```python
from build123d import *

# Parameters (mm, degrees)
F1_DEPTH = 50.8
F2_R     = 50.8
F3_R     = 5.08


with BuildPart() as f1:
    # F0 (on Top) → F1 (new body)
    with BuildSketch(Plane.XY):
        Polygon((836.6125, 0), (-836.6125, 0), (-836.6125, -147.6375), (-582.6125, -655.6375), (582.6125, -655.6375), (836.6125, -147.6375), align=None)
    extrude(amount=-F1_DEPTH)

    # F2
    f2_edges = [f1.edges().sort_by_distance(p)[0] for p in [
        (-836.6125, -147.6375, -25.4),
        (-582.6125, -655.6375, -25.4),
        (582.6125, -655.6375, -25.4),
        (836.6125, -147.6375, -25.4),
    ]]
    fillet(f2_edges, radius=F2_R)

    # F3
    f3_edges = [f1.edges().sort_by_distance(p)[0] for p in [
        (836.6125, 0, -25.4),
        (-836.6125, 0, -25.4),
    ]]
    fillet(f3_edges, radius=F3_R)


solid = f1.part
```
Here's how the part is built. I have some questions about the finished solid (model axes, mm). Coordinates: 2 decimals unless noted, no trailing zeros. Order: outer loops, then holes, each group sorted by start corner. A loop starts at its lowest first (then second) coordinate and runs counter-clockwise, first axis right, second up.
1) I need wall thicknesses on line 1 (X direction, y = -137, z = -15.5); line 2 (X direction, y = -367, z = -37.5); line 3 (Y direction, x = 663.5, z = -19.5). Which ranges of each line are inside material? Lowest first, please.
2) Imagine slicing it at A-A on z = -19. List the corners of the cut face in (x, y) for me, and give its area (3 significant figures).
3) Imagine slicing it at B-B on y = -557. List the corners of the cut face in (x, z) for me, and give its area (3 significant figures).
4) Will these pins go through, and if not, where does the flat tip stop? pin 1 (4 mm diameter, centred on y = -371, z = -26.5, fed in from +X); pin 2 (1.5 mm diameter, centred on y = -383.5, z = -44.5, fed in from +X).
5) Imagine slicing it at C-C on x = -630.5. List the corners of the cut face in (y, z) for me, and give its area (3 significant figures).
Response values:
1. line 1: x = -836.59 to 836.59
1. line 2: x = -726.93 to 726.93
1. line 3: y = -493.86 to 0
2. outline: (-836.61, -135.65) arc R50.8 ccw to (-831.25, -158.36) - (-596.65, -627.56) arc R50.8 ccw to (-551.22, -655.64) - (551.22, -655.64) arc R50.8 ccw to (596.65, -627.56) - (831.25, -158.36) arc R50.8 ccw to (836.61, -135.65) - (836.61, -5.08) arc R5.08 ccw to (831.53, 0) - (-831.53, 0) arc R5.08 ccw to (-836.61, -5.08) - close
2. area: 968,000 mm2
3. outline: (-631.93, -50.8) - (631.93, -50.8) - (631.93, 0) - (-631.93, 0) - close
3. area: 64,200 mm2
4. pin 1: stops at x = 725.93
4. pin 2: stops at x = 719.06
5. outline: (-559.86, -50.8) - (0, -50.8) - (0, 0) - (-559.86, 0) - close
5. area: 28,400 mm2
